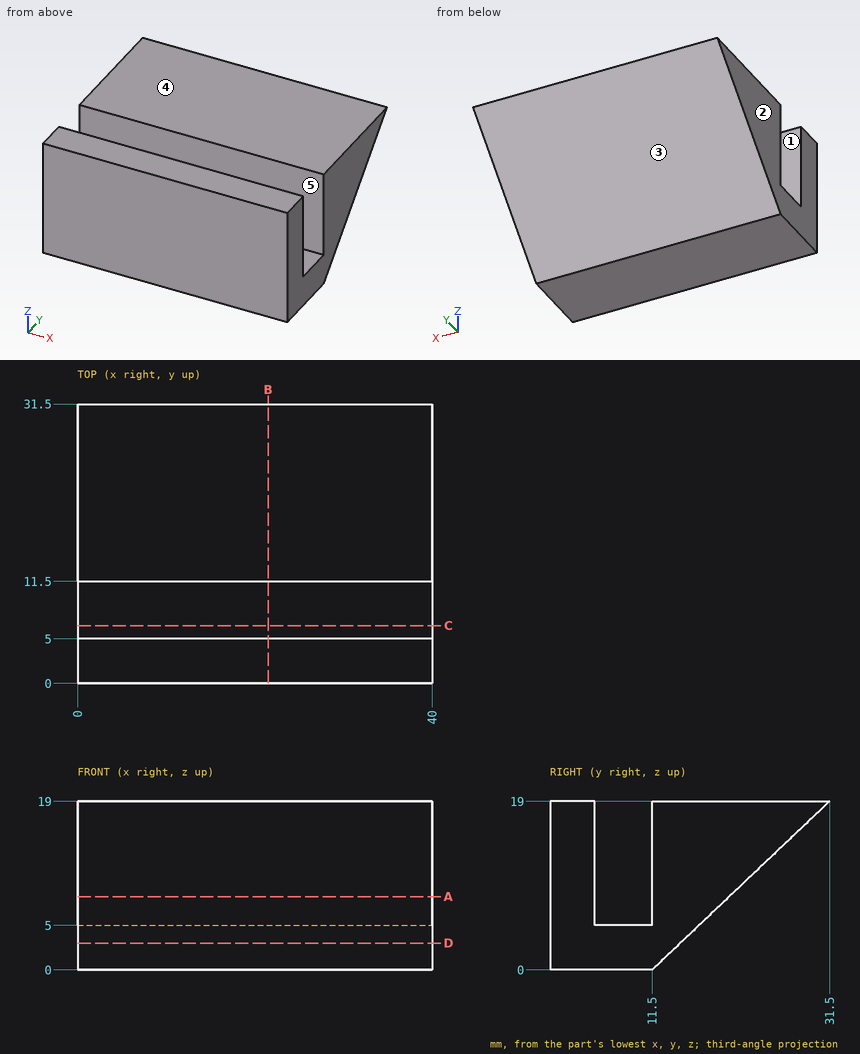
Geometry: see drawing. Coordinates: mm, zero at the bounding-box minimum. A direction names the side the tool comes from. Round coordinates to 2 decimals unless told otherwise and drop trailing zeros. Loops run counter-clockwise (first coordinate to the right, second up) from the corner with the lowest first, then second, coordinate; pieces in that order, holes last. Notation, with made-up numbers: (62, 33.25) - (72, 33.25) arc R13 ccw to (72, 41.25) - close; hole circle Ø7 at (61, 58.25). An arc over 180 degrees is marked (long way). One line per item, written item: value. Start each with the question number.
(1) Ray query, line 1 (Z direction, x = 5, y = 10); line 2 (Y direction, x = 9, z = 6.25); line 3 (Y direction, x = 18, z = 11.25). Return the intervals inside material, ascending. Write a range as [from, to].
(2) Section D-D, the plane z = 3. Return loops of the section in (x, y).
(3) Section C-C, the plane y = 6.5. Return loops of the section in (x, z).
(4) Access query for the marked faces 1 and 2. Directions: +Z, -Z, +X, -X, +Y, -Y. A direction counts if a zero-diameter tool reaches every point of the face in a straight line with its end or side. Return the directions, or none.
(5) Section B-B, the plane x = 21.5. Return loops of the section in (y, z), plus the area to 4 significant figures.
(6) Draft query along Y for the marked faces 3, 4 and 5. Return one class per face: +Y half, -Y half, draft (parallel to the pull), parting line (faces both ways), or undercut.
(7) Contact query for flat-ended pins moving along their axis: P1, Ø3, axis at x = 35, y = 22, coming from the -Z side; P2, Ø10, axis at x = 26.5, z = 6.5, coming from the +Y side; P3, Ø11, axis at x = 24.5, z = 13, coming from the +Y side. Output: stop coordinate, or through.
(8) Section A-A, the plane z = 8.25. Return loops of the section in (x, y), plus the area to 3 significant figures.
Results below:
1. line 1: [0, 5]
1. line 2: [0, 5], [11.5, 18.08]
1. line 3: [0, 5], [11.5, 23.34]
2. outline: (0, 0) - (40, 0) - (40, 14.66) - (0, 14.66) - close
3. outline: (0, 0) - (40, 0) - (40, 5) - (0, 5) - close
4. face 1: +Z, +X, -X
4. face 2: +Z, -Z, -X, +Y, -Y
5. outline: (0, 0) - (11.5, 0) - (31.5, 19) - (11.5, 19) - (11.5, 5) - (5, 5) - (5, 19) - (0, 19) - close
5. area: 317.5 mm^2
6. face 3: +Y half
6. face 4: draft
6. face 5: undercut
7. P1: z = 8.55
7. P2: y = 23.61
7. P3: y = 30.97
8. outline: (0, 0) - (40, 0) - (40, 5) - (0, 5) - close; (0, 11.5) - (40, 11.5) - (40, 20.18) - (0, 20.18) - close
8. area: 547 mm^2
